Work out the finished part from the listing and answer in its coordinate system (mm). A direction names the side the tool comes from. Round coordinates to 2 decimals unless told otherwise and drop trailing zeros. Loops run counter-clockwise (first coordinate to the right, second up) from the corner with the lowest first, then second, coordinate; pieces in that order, holes last. Notation, with made-up numbers: (-36, 48.25) -> (-2, 48.25) arc R30 ccw to (-2, 73.25) -> close; hole circle Ø11 at (52.25, 17.5). An arc over 180 degrees is marked (long way). Write item = value, one per line. Start each with the question number.
```python
from build123d import *

# Parameters (mm, degrees)
SKETCH_1_R          = 1.4
SKETCH_1_W          = 40
SKETCH_1_H          = 50
EXTRUDE_1_DEPTH     = 3
SKETCH_2_R          = 1.4
EXTRUDE_2_DEPTH     = 7
SKETCH_3_R          = 1.4
CUT_EXTRUDE_1_DEPTH = 7
SKETCH_4_R          = 3
CUT_EXTRUDE_2_DEPTH = 3
FILLET_1_R          = 1
FILLET_2_R          = 2
FILLET_3_R          = 5


with BuildPart() as part:
    # 草图1 → 凸台-拉伸1 (new body)
    with BuildSketch(Plane(origin=(0, 0, 0), x_dir=(1, 0, 0), z_dir=(0, 1, 0))):
        Polygon((-40, 22), (-40, -31), (-25.773502692, -31), (-20, -41), (20, -41), (25.773502692, -31), (40, -31), (50, -21), (50, 22), (38, 34), (-28, 34), align=None)
        with Locations(Location((-35.75, 14, 0), (0, 0, 270))):
            Circle(SKETCH_1_R, mode=Mode.SUBTRACT)
        with Locations(Location((35.75, 14, 0), (0, 0, 270))):
            Circle(SKETCH_1_R, mode=Mode.SUBTRACT)
        with Locations(Location((-35.75, -14, 0), (0, 0, 270))):
            Circle(SKETCH_1_R, mode=Mode.SUBTRACT)
        with Locations(Location((45.75, 19, 0), (0, 0, 270))):
            Circle(SKETCH_1_R, mode=Mode.SUBTRACT)
        with Locations(Location((45.75, -9, 0), (0, 0, 270))):
            Circle(SKETCH_1_R, mode=Mode.SUBTRACT)
        with Locations(Location((-25.75, 19, 0), (0, 0, 270))):
            Circle(SKETCH_1_R, mode=Mode.SUBTRACT)
        with Locations((5, 1)):
            Rectangle(SKETCH_1_W, SKETCH_1_H, mode=Mode.SUBTRACT)
    extrude(amount=EXTRUDE_1_DEPTH)

    # 草图2 → 凸台-拉伸2 (add)
    # profile 1 of 2: a face of its own
    with BuildSketch(Plane(origin=(0, 3, 0), x_dir=(1, 0, 0), z_dir=(0, 1, 0))):
        Polygon((-19, 34), (-19, 0.773502692), (-25.773502692, -6), (-25.773502692, -31), (-40, -31), (-40, 22), (-28, 34), align=None)
        with Locations(Location((-35.75, -14, 0), (0, 0, 270))):
            Circle(SKETCH_2_R, mode=Mode.SUBTRACT)
        with Locations(Location((-35.75, 14, 0), (0, 0, 270))):
            Circle(SKETCH_2_R, mode=Mode.SUBTRACT)
        with Locations(Location((-25.75, 19, 0), (0, 0, 270))):
            Circle(SKETCH_2_R, mode=Mode.SUBTRACT)
    # profile 2 of 2: a face of its own
    with BuildSketch(Plane(origin=(0, 3, 0), x_dir=(1, 0, 0), z_dir=(0, 1, 0))):
        Polygon((29, 34), (29, 15), (40, 4), (40, -31), (50, -21), (50, 22), (38, 34), align=None)
        with Locations(Location((45.75, -9, 0), (0, 0, 270))):
            Circle(SKETCH_2_R, mode=Mode.SUBTRACT)
        with Locations(Location((45.75, 19, 0), (0, 0, 270))):
            Circle(SKETCH_2_R, mode=Mode.SUBTRACT)
        with Locations(Location((35.75, 14, 0), (0, 0, 270))):
            Circle(SKETCH_2_R, mode=Mode.SUBTRACT)
    extrude(amount=EXTRUDE_2_DEPTH)

    # 草图3 → 切除-拉伸1 (cut)
    with BuildSketch(Plane(origin=(0, 0, -34), x_dir=(-1, 0, 0), z_dir=(0, 0, -1))):
        with Locations((-33, 6)):
            Circle(SKETCH_3_R)
        with Locations((23, 6)):
            Circle(SKETCH_3_R)
    extrude(amount=-CUT_EXTRUDE_1_DEPTH, mode=Mode.SUBTRACT)

    # 草图4 → 切除-拉伸2 (cut)
    with BuildSketch(Plane.XZ):
        with Locations((46, 21)):
            Circle(SKETCH_4_R)
        with Locations(Location((46, 1, 0), (0, 0, 270))):
            Circle(SKETCH_4_R)
        with Locations(Location((32, 20, 0), (0, 0, 270))):
            Circle(SKETCH_4_R)
        with Locations(Location((32, 2, 0), (0, 0, 270))):
            Circle(SKETCH_4_R)
        with Locations((13, 25)):
            Circle(SKETCH_4_R)
    extrude(amount=-CUT_EXTRUDE_2_DEPTH, mode=Mode.SUBTRACT)

    # 圆角1
    # the kernel refuses this fillet: 1 mm, written as the material it takes off along each edge
    with BuildSketch(Plane(origin=(47.292893219, 3, 23.707106781), x_dir=(-0.9977260233446211, 0, 0.0674001657336884), z_dir=(0, -1, 0))) as fillet_1_piece_1:
        with BuildLine():
            CenterArc((2.584152116, -0.929364034), FILLET_1_R, 111.664104493, 117.20057038)
            Line((1.926312394, -1.682521985), (1.913155599, -1.697585144))
            Line((1.913155599, -1.697585144), (-0.013156794, -0.015063159))
            Line((-0.013156794, -0.015063159), (0.007383292, 0.018587281))
            ThreePointArc((0.007383292, 0.018587281), (1.107493764, -0.191907899), (2.207604236, 0.018587281))
            Line((2.207604236, 0.018587281), (2.214987528, 0))
        make_face()
    extrude(amount=9.394118228, mode=Mode.SUBTRACT)
    with BuildSketch(Plane(origin=(48.707106781, 3, 22.292893219), x_dir=(0.09729861673044447, 0, -0.9952552331851072), z_dir=(0, -1, 0))) as fillet_1_piece_2:
        with BuildLine():
            CenterArc((2.387842326, 0.940019638), FILLET_1_R, 167.235610317, 82.819244219)
            Line((1.412555464, 1.16096202), (1.393049727, 1.165380868))
            ThreePointArc((1.393049727, 1.165380868), (0.693578708, 0.595932055), (-0.012699024, 0.015451045))
            Line((-0.012699024, 0.015451045), (0.006822407, -0.018800393))
            ThreePointArc((0.006822407, -0.018800393), (1.023360997, 0.159941087), (2.039899587, -0.018800393))
            Line((2.039899587, -0.018800393), (2.046721994, 0))
        make_face()
    extrude(amount=8.116804984, mode=Mode.SUBTRACT)
    with BuildSketch(Plane(origin=(10.171572875, 5.928932188, 24), x_dir=(-1, 0, 0), z_dir=(0, -1, 0))) as fillet_1_piece_3:
        with BuildLine():
            CenterArc((1.171572875, -1), FILLET_1_R, 90, 90)
            Line((0.171572875, -1), (0.151572875, -1))
            ThreePointArc((0.151572875, -1), (0.108656583, -0.496076103), (-0.018856181, -0.006666667))
            Line((-0.018856181, -0.006666667), (0, 0.02))
            Line((0, 0.02), (1.171572875, 0.02))
            Line((1.171572875, 0.02), (1.171572875, 0))
        make_face()
    extrude(amount=8.857864376, mode=Mode.SUBTRACT)
    with BuildSketch(Plane(origin=(15.828427125, 5.928932188, 24), x_dir=(0.1691019787257596, 0, 0.9855985596534894), z_dir=(0, -1, 0))) as fillet_1_piece_4:
        with BuildLine():
            CenterArc((1.183713851, -0.98559856), FILLET_1_R, 99.735610317, 90)
            Line((0.198115291, -1.154700538), (0.17840332, -1.158082578))
            Line((0.17840332, -1.158082578), (-0.019711971, -0.00338204))
            Line((-0.019711971, -0.00338204), (0.00338204, 0.019711971))
            ThreePointArc((0.00338204, 0.019711971), (0.507305936, -0.023204321), (1.011229833, 0.019711971))
            Line((1.011229833, 0.019711971), (1.014611872, 0))
        make_face()
    extrude(amount=8.857864376, mode=Mode.SUBTRACT)

    # 圆角2
    fillet_2_edges = [part.edges().sort_by_distance(p)[0] for p in [
        (25.773502692, 1.5, 31),
        (20, 1.5, 41),
        (-20, 1.5, 41),
        (-25.773502692, 1.5, 31),
    ]]
    fillet(fillet_2_edges, radius=FILLET_2_R)

    # 圆角3
    fillet_3_edges = [part.edges().sort_by_distance(p)[0] for p in [
        (-15, 1.5, -26),
        (-15, 1.5, 24),
        (25, 1.5, 24),
        (25, 1.5, -26),
    ]]
    fillet(fillet_3_edges, radius=FILLET_3_R)


solid = part.part
```
Item 1: The mould has two halves that part along X. Classify faces 5 (the flat face through (50, 5, 0)), 6 (the flat face through (42, 10, -9)), 7 (the flat face through (-25.774, 6, 18)): pulls with the +X half, pulls with the -X half, needs draft (parallel to the pull), parting line crosses it, or undercut.
Item 2: Section A-A (z = -14) is taken. Determine the outline of the cut face in (x, y).
Item 3: A tool of negligible diameter and unlimited length cuts with its end or side. For faces 1 (the flat face through (-15, 1, -1)), 2 (the flat face through (46, 3, 21)), 3 (the flat face through (34, 6, -10)), 4 (the flat face through (29, 6, -25)), from which of +Z, -Z, +X, -X, +Y, -Y can it reach the whole face along a straight path? Write none if from no direction.
Item 4: Section D-D (z = 14) is taken. Determine the outline of the cut face in (x, y), then the cut area to 3 significant figures.
Item 5: Section C-C (x = 13) is taken. Determine the outline of the cut face in (y, z).
Item 6: Find the intervals of material crossed by line 1 along X through (y, z) = (4.75, -19); line 2 along X through (y, z) = (4, -14); line 3 along Z through (x, y) = (2, 0.5), in increasing order. Write a range as [from, to].
Item 7: Section B-B (z = -25) is taken. Determine the outline of the cut face in (x, y), then the cut area to 3 significant figures.
Item 8: Flat-ended cylindrical pins translate along their axes: pin 1 (2.5 mm diameter, centred on x = 45.75, z = 9, fed in from +Y); pin 2 (4.5 mm diameter, centred on x = 33, y = 6, fed in from +Z); pin 3 (3.5 mm diameter, centred on y = 8, z = -28, fed in from -X). Find the tip coordinate at first contact, or state that the pin passes through.
Worked answers:
q1.face_5 = pulls with the +X half
q1.face_6 = needs draft
q1.face_7 = undercut
q2.outline = (-40, 0) -> (-37.15, 0) -> (-37.15, 10) -> (-40, 10) -> close; (-34.35, 0) -> (-15, 0) -> (-15, 3) -> (-19, 3) -> (-19, 10) -> (-34.35, 10) -> close; (25, 0) -> (34.35, 0) -> (34.35, 10) -> (30, 10) -> (30, 3) -> (25, 3) -> close; (37.15, 0) -> (50, 0) -> (50, 10) -> (37.15, 10) -> close
q3.face_1 = +Y, -Y
q3.face_2 = -Y
q3.face_3 = +Z, +Y
q3.face_4 = +Z, -Z, +Y
q4.outline = (-40, 0) -> (-37.15, 0) -> (-37.15, 10) -> (-40, 10) -> close; (-34.35, 0) -> (-15, 0) -> (-15, 3) -> (-25.77, 3) -> (-25.77, 10) -> (-34.35, 10) -> close; (25, 0) -> (50, 0) -> (50, 10) -> (40, 10) -> (40, 3) -> (25, 3) -> close
q4.area = 292 mm2
q5.outline = (0, -34) -> (3, -34) -> (3, -26) -> (0, -26) -> close; (0, 28) -> (3, 28) -> (3, 41) -> (0, 41) -> close
q6.line_1 = [-40, -27.15], [-24.35, -19], [29, 44.35], [47.15, 50]
q6.line_2 = [-40, -37.15], [-34.35, -19], [30, 34.35], [37.15, 50]
q6.line_3 = [-34, -26], [24, 41]
q7.outline = (-37, 0) -> (-13, 0) -> (-13, 3) -> (-19, 3) -> (-19, 10) -> (-37, 10) -> close; (23, 0) -> (47, 0) -> (47, 10) -> (29, 10) -> (29, 3) -> (23, 3) -> close
q7.area = 396 mm2
q8.pin_1 = through
q8.pin_2 = -8.75
q8.pin_3 = -35.75
